```python
from build123d import *

# Parameters (mm, degrees)
F0_W     = 550
F0_H     = 270
F1_DEPTH = 10
F3_DEPTH = 6
F2_R     = 2.5
F4_DEPTH = 25
F5_R     = 5


with BuildPart() as f1:
    # F0 (on Top) → F1 (new body)
    with BuildSketch(Plane.XY):
        with Locations((275, -135)):
            Rectangle(F0_W, F0_H)
    extrude(amount=-F1_DEPTH)

    # F2 (on face) → F3 (cut)
    with BuildSketch(Plane.XY):
        with BuildLine():
            ThreePointArc((93.8406279725, -17.4723188671), (96.3763447636, -34.89397928), (100.5834584289, -51.9891337337))
            ThreePointArc((100.5834584289, -51.9891337337), (101.702824577, -52.2182469254), (102.8172889589, -52.4701250099))
            ThreePointArc((102.8172889589, -52.4701250099), (98.4454239564, -35.0497029669), (95.8313903025, -17.2803153631))
            Line((95.8313903025, -17.2803153631), (93.8406279725, -17.4723188671))
        make_face()
        with BuildLine():
            ThreePointArc((36.6062109858, -22.9924196081), (40.2678425285, -47.5506492992), (46.4524007703, -71.5977994519))
            ThreePointArc((46.4524007703, -71.5977994519), (70.8084957225, -54.3138897804), (100.5834584289, -51.9891337337))
            ThreePointArc((100.5834584289, -51.9891337337), (96.3763447636, -34.89397928), (93.8406279725, -17.4723188671))
            Line((93.8406279725, -17.4723188671), (36.6062109858, -22.9924196081))
        make_face()
        with BuildLine():
            ThreePointArc((26.1547087534, -24.0004380043), (30.8880481953, -53.9384370008), (39.2095922874, -83.0835942334))
            ThreePointArc((39.2095922874, -83.0835942334), (42.4819606163, -77.1205988593), (46.4524007703, -71.5977994519))
            ThreePointArc((46.4524007703, -71.5977994519), (40.2678425285, -47.5506492992), (36.6062109858, -22.9924196081))
            Line((36.6062109858, -22.9924196081), (26.1547087534, -24.0004380043))
        make_face()
        with BuildLine():
            ThreePointArc((39.2095922874, -83.0835942334), (41.3696850637, -135.0845918815), (85.359218008, -162.8998889056))
            ThreePointArc((85.359218008, -162.8998889056), (58.5731428007, -125.1375862115), (39.2095922874, -83.0835942334))
        make_face()
        with BuildLine():
            ThreePointArc((39.2095922874, -83.0835942334), (58.5731428007, -125.1375862115), (85.359218008, -162.8998889056))
            ThreePointArc((85.359218008, -162.8998889056), (92.159689712, -163.0387878421), (98.9269281749, -162.353082441))
            ThreePointArc((98.9269281749, -162.353082441), (67.6630708031, -119.8818075906), (46.4524007703, -71.5977994519))
            ThreePointArc((46.4524007703, -71.5977994519), (42.4819606163, -77.1205988593), (39.2095922874, -83.0835942334))
        make_face()
        with BuildLine():
            ThreePointArc((46.4524007703, -71.5977994519), (67.6630708031, -119.8818075906), (98.9269281749, -162.353082441))
            ThreePointArc((98.9269281749, -162.353082441), (126.0574308053, -149.8675419291), (142.9268949098, -125.2225814773))
            ThreePointArc((142.9268949098, -125.2225814773), (117.4412479589, -91.100162762), (100.5834584289, -51.9891337337))
            ThreePointArc((100.5834584289, -51.9891337337), (70.8084957225, -54.3138897804), (46.4524007703, -71.5977994519))
        make_face()
        with BuildLine():
            ThreePointArc((100.5834584289, -51.9891337337), (117.4412479589, -91.100162762), (142.9268949098, -125.2225814773))
            ThreePointArc((142.9268949098, -125.2225814773), (143.2867819227, -124.1381669965), (143.6244940218, -123.0466433063))
            ThreePointArc((143.6244940218, -123.0466433063), (119.1726628165, -90.0990620723), (102.8172889589, -52.4701250099))
            ThreePointArc((102.8172889589, -52.4701250099), (101.702824577, -52.2182469254), (100.5834584289, -51.9891337337))
        make_face()
        with BuildLine():
            ThreePointArc((102.8172889589, -52.4701250099), (119.1726628165, -90.0990620723), (143.6244940218, -123.0466433063))
            ThreePointArc((143.6244940218, -123.0466433063), (145.375436454, -115.11981647), (145.9631920321, -107.023216784))
            ThreePointArc((145.9631920321, -107.023216784), (133.8730301026, -72.2467564476), (102.8172889589, -52.4701250099))
        make_face()
        with BuildLine():
            ThreePointArc((142.9268949098, -125.2225814773), (165.4491613095, -145.3362093293), (190.9870540226, -161.4491403142))
            Line((190.9870540226, -161.4491403142), (191.9102732092, -159.6749739371))
            ThreePointArc((191.9102732092, -159.6749739371), (166.2146946142, -143.4076613439), (143.6244940218, -123.0466433063))
            ThreePointArc((143.6244940218, -123.0466433063), (143.2867819227, -124.1381669965), (142.9268949098, -125.2225814773))
        make_face()
        with BuildLine():
            ThreePointArc((98.9269281749, -162.353082441), (129.5126452175, -190.2463655327), (164.4445024089, -212.4564236553))
            Line((164.4445024089, -212.4564236553), (190.9870540226, -161.4491403142))
            ThreePointArc((190.9870540226, -161.4491403142), (165.4491613095, -145.3362093293), (142.9268949098, -125.2225814773))
            ThreePointArc((142.9268949098, -125.2225814773), (126.0574308053, -149.8675419291), (98.9269281749, -162.353082441))
        make_face()
        with BuildLine():
            ThreePointArc((85.359218008, -162.8998889056), (119.6639725539, -195.884452107), (159.5976016794, -221.7707971349))
            Line((159.5976016794, -221.7707971349), (164.4445024089, -212.4564236553))
            ThreePointArc((164.4445024089, -212.4564236553), (129.5126452175, -190.2463655327), (98.9269281749, -162.353082441))
            ThreePointArc((98.9269281749, -162.353082441), (92.159689712, -163.0387878421), (85.359218008, -162.8998889056))
        make_face()
    extrude(amount=-F3_DEPTH, mode=Mode.SUBTRACT)

    # F2 (on face) → F4 (cut)
    with BuildSketch(Plane.XY):
        with BuildLine():
            ThreePointArc((17.5, -255), (13.232233047, -253.232233047), (15, -257.5))
            ThreePointArc((15, -257.5), (16.767766953, -256.767766953), (17.5, -255))
        make_face()
        with Locations((15, -15)):
            Circle(F2_R)
        with BuildLine():
            ThreePointArc((537.5, -15), (536.767766953, -13.232233047), (535, -12.5))
            ThreePointArc((535, -12.5), (533.232233047, -16.767766953), (537.5, -15))
        make_face()
        with Locations((535, -255)):
            Circle(F2_R)
    extrude(amount=-F4_DEPTH, mode=Mode.SUBTRACT)

    # F5
    f5_edges = [f1.edges().sort_by_distance(p)[0] for p in [
        (102.817289, -52.470125, -3),
        (143.624494, -123.046643, -3),
        (85.359218, -162.899889, -3),
        (39.209592, -83.083594, -3),
    ]]
    fillet(f5_edges, radius=F5_R)


solid = f1.part
```
Could you check a few things on this model? Use its own coordinates, in mm. A direction names the side the tool comes from. Coordinates: 2 decimals unless noted, no trailing zeros. Order: outer loops, then holes, each group sorted by start corner. A loop starts at its lowest first (then second) coordinate and runs counter-clockwise, first axis right, second up. Notation, with made-up numbers: M 46.5,-15 L 82.5,-15 A5 cw 82.5,-7 Z; hole C 73.25,86 d10. An arc over 180 degrees is marked long. Use a Markdown table: item, result. Add a question column.
Q1. I'm going to push a flat-ended pin straight in: pin 1 (4 mm diameter, centred on x = 535, y = -15, fed in from +Z). Where does the tip first touch, or does it pass through?
Q2. Which directions (+Z, -Z, +X, -X, +Y, -Y) give clear straight access to the entire face, cutting with the end or side of a thin tool? Please do faces 5 (the flat face through (108, -118, -6)), 6 (the flat face through (271, -270, -5)).
Q3. I want a section at B-B on x = 61.5. List the corners of the cut face in (y, z) for me.
Q4. I want a section at A-A on z = -2. Give the number of separate pieces and of enclosed holes in the cut face, then the cut area to 3 significant figures.
Q5. We'd pull the mould along X, two halves only. Please class faces 1 (the cylindrical face through (119.925, -196.091, -2.958)), 2 (the cylindrical face through (41.01, -134.45, -2.96)), 3 (the flat face through (550, -137, -5)), 4 (the flat face through (271, 0, -5)): pulls with the +X half, pulls with the -X half, needs draft (parallel to the pull), parting line crosses it, or undercut.
Q6. I want a section at C-C on y = -174. List the corners of the cut face in (x, z) for me.
Q7. If I drill on L1, parallel to Y at x = 535, z = -4; L2, parallel to X at y = -255, z = -2.75; L3, parallel to X at y = -108.5, z = -3, over which ranges is the centre line in solid material (lowest first)?
Checked values:
| question | item | result |
|---|---|---|
| 1 | pin 1 | through |
| 2 | face 5 | +Z |
| 2 | face 6 | +Z, -Z, +X, -X, -Y |
| 3 | outline | M -270,-10 L 0,-10 L 0,0 L -20.59,0 L -20.59,-6 L -155.36,-6 L -155.36,0 L -270,0 Z |
| 4 | separate pieces | 1 |
| 4 | enclosed holes | 5 |
| 4 | area | 131,000 mm² |
| 5 | face 1 | undercut |
| 5 | face 2 | undercut |
| 5 | face 3 | pulls with the +X half |
| 5 | face 4 | needs draft |
| 6 | outline | M 0,-10 L 550,-10 L 550,0 L 184.46,0 L 184.46,-6 L 95.49,-6 L 95.49,0 L 0,0 Z |
| 7 | L1 | -270 to -257.5, -252.5 to -17.5, -12.5 to 0 |
| 7 | L2 | 0 to 12.5, 17.5 to 532.5, 537.5 to 550 |
| 7 | L3 | 0 to 33.86, 145.94 to 550 |
